```python
from build123d import *

# Parameters (mm, degrees)
SKETCH1_R           = 7.5
BOSS_EXTRUDE1_DEPTH = 46
SKETCH2_W           = 15
SKETCH2_H           = 15
BOSS_EXTRUDE2_DEPTH = 10
BOSS_EXTRUDE3_DEPTH = 15
CUT_EXTRUDE4_DEPTH  = 64.263338514
SKETCH6_R           = 6
CUT_EXTRUDE5_DEPTH  = 64.263338514
SKETCH7_R           = 6
CUT_EXTRUDE6_DEPTH  = 5
CUT_EXTRUDE7_START  = -5
CUT_EXTRUDE7_DEPTH  = 5
SKETCH11_R          = 3.25
SKETCH11_R_2        = 2.25
BOSS_EXTRUDE4_DEPTH = 2.5
BOSS_EXTRUDE5_DEPTH = 2.5


with BuildPart() as part:
    # Sketch1 → Boss-Extrude1 (new body)
    with BuildSketch(Plane(origin=(0, 0, 0), x_dir=(1, 0, 0), z_dir=(0, 1, 0))):
        with Locations(Location((0, 0, 0), (0, 0, 270))):
            Circle(SKETCH1_R)
    extrude(amount=BOSS_EXTRUDE1_DEPTH)

    # Sketch2 → Boss-Extrude2 (add)
    with BuildSketch(Plane.XZ):
        Rectangle(SKETCH2_W, SKETCH2_H)
    extrude(amount=BOSS_EXTRUDE2_DEPTH)

    # Sketch4 → Boss-Extrude3 (add)
    with BuildSketch(Plane(origin=(0, 46, 0), x_dir=(1, 0, 0), z_dir=(0, 1, 0))):
        Polygon((0, 7.5), (7.5, 7.5), (7.5, -7.5), (-7.5, -7.5), (-7.5, 7.5), align=None)
    extrude(amount=BOSS_EXTRUDE3_DEPTH)

    # Sketch5 → Cut-Extrude4 (cut, through all)
    with BuildSketch(Plane.ZY.offset(7.5)):
        with BuildLine():
            ThreePointArc((-7.5, 53.5), (-5.303300859, 58.803300859), (0, 61))
            Line((0, 61), (-7.5, 61))
            Line((-7.5, 61), (-7.5, 53.5))
        make_face()
        with BuildLine():
            Line((7.5, 61), (0, 61))
            ThreePointArc((0, 61), (5.303300859, 58.803300859), (7.5, 53.5))
            Line((7.5, 53.5), (7.5, 61))
        make_face()
    extrude(amount=-CUT_EXTRUDE4_DEPTH, mode=Mode.SUBTRACT)

    # Sketch6 → Cut-Extrude5 (cut, through all)
    with BuildSketch(Plane.ZY.offset(7.5)):
        with Locations((0, 53.5)):
            Circle(SKETCH6_R)
    extrude(amount=-CUT_EXTRUDE5_DEPTH, mode=Mode.SUBTRACT)

    # Sketch7 → Cut-Extrude6 (cut)
    # profile 1 of 4: a face of its own
    with BuildSketch(Plane.ZY.offset(7.5)):
        with BuildLine():
            ThreePointArc((0, 46), (-5.303300859, 48.196699141), (-7.5, 53.5))
            Line((-7.5, 53.5), (-7.5, 46))
            Line((-7.5, 46), (0, 46))
        make_face()
    # profile 2 of 4: a face of its own
    with BuildSketch(Plane.ZY.offset(7.5)):
        with BuildLine():
            Line((7.5, 46), (7.5, 53.5))
            ThreePointArc((7.5, 53.5), (5.303300859, 48.196699141), (0, 46))
            Line((0, 46), (7.5, 46))
        make_face()
    # profile 3 of 4: a face of its own
    with BuildSketch(Plane.ZY.offset(7.5)):
        with BuildLine():
            ThreePointArc((7.5, 53.5), (0, 61), (-7.5, 53.5))
            ThreePointArc((-7.5, 53.5), (-5.303300859, 48.196699141), (0, 46))
            ThreePointArc((0, 46), (5.303300859, 48.196699141), (7.5, 53.5))
        make_face()
        with Locations((0, 53.5)):
            Circle(SKETCH7_R, mode=Mode.SUBTRACT)
    # profile 4 of 4: a face of its own
    with BuildSketch(Plane.ZY.offset(7.5)):
        with Locations((0, 53.5)):
            Circle(SKETCH7_R)
    extrude(amount=-CUT_EXTRUDE6_DEPTH, mode=Mode.SUBTRACT)

    # Sketch10 → Cut-Extrude7 (cut)
    with BuildSketch(Plane(origin=(7.5, 0, 0), x_dir=(0, 0, -1), z_dir=(1, 0, 0)).offset(CUT_EXTRUDE7_START)):
        with BuildLine():
            Line((7.5, 53.5), (6, 53.5))
            ThreePointArc((6, 53.5), (0, 47.5), (-6, 53.5))
            Line((-6, 53.5), (-7.5, 53.5))
            Line((-7.5, 53.5), (-7.5, 46))
            Line((-7.5, 46), (0, 46))
            Line((0, 46), (7.5, 46))
            Line((7.5, 46), (7.5, 53.5))
        make_face()
        with BuildLine():
            ThreePointArc((-6, 53.5), (0, 59.5), (6, 53.5))
            Line((6, 53.5), (7.5, 53.5))
            ThreePointArc((7.5, 53.5), (0, 61), (-7.5, 53.5))
            Line((-7.5, 53.5), (-6, 53.5))
        make_face()
    extrude(amount=CUT_EXTRUDE7_DEPTH, mode=Mode.SUBTRACT)

    # Sketch11 → Boss-Extrude4 (add, symmetric)
    # profile 1 of 3: a face of its own
    with BuildSketch(Plane(origin=(0, 0, 0), x_dir=(-1, 0, 0), z_dir=(0, 0, -1))):
        with BuildLine():
            Line((7.5, -1.75), (7.5, -5))
            ThreePointArc((7.5, -5), (8.451902961, -2.701902961), (10.75, -1.75))
            Line((10.75, -1.75), (7.5, -1.75))
        make_face()
    # profile 2 of 3: a face of its own
    with BuildSketch(Plane(origin=(0, 0, 0), x_dir=(-1, 0, 0), z_dir=(0, 0, -1))):
        with BuildLine():
            Line((7.5, -5), (7.5, -8.25))
            Line((7.5, -8.25), (10.75, -8.25))
            ThreePointArc((10.75, -8.25), (8.451902961, -7.298097039), (7.5, -5))
        make_face()
    # profile 3 of 3: a face of its own
    with BuildSketch(Plane(origin=(0, 0, 0), x_dir=(-1, 0, 0), z_dir=(0, 0, -1))):
        with Locations((10.75, -5)):
            Circle(SKETCH11_R)
        with Locations((10.75, -5)):
            Circle(SKETCH11_R_2, mode=Mode.SUBTRACT)
    extrude(amount=BOSS_EXTRUDE4_DEPTH, both=True)

    # Sketch12 → Boss-Extrude5 (add, symmetric)
    with BuildSketch(Plane(origin=(0, 0, 0), x_dir=(-1, 0, 0), z_dir=(0, 0, -1))):
        with BuildLine():
            Line((-7.5, -8.25), (-7.5, -5))
            ThreePointArc((-7.5, -5), (-8.451902961, -7.298097039), (-10.75, -8.25))
            Line((-10.75, -8.25), (-7.5, -8.25))
        make_face()
        with BuildLine():
            Line((-7.5, -5), (-7.5, -1.75))
            Line((-7.5, -1.75), (-10.75, -1.75))
            ThreePointArc((-10.75, -1.75), (-8.451902961, -2.701902961), (-7.5, -5))
        make_face()
        with BuildLine():
            ThreePointArc((-7.5, -5), (-8.451902961, -2.701902961), (-10.75, -1.75))
            Line((-10.75, -1.75), (-10.75, -2.75))
            ThreePointArc((-10.75, -2.75), (-9.159009742, -3.409009742), (-8.5, -5))
            Line((-8.5, -5), (-7.5, -5))
        make_face()
        with BuildLine():
            ThreePointArc((-10.75, -8.25), (-8.451902961, -7.298097039), (-7.5, -5))
            Line((-7.5, -5), (-8.5, -5))
            ThreePointArc((-8.5, -5), (-9.159009742, -6.590990258), (-10.75, -7.25))
            Line((-10.75, -7.25), (-10.75, -8.25))
        make_face()
        with BuildLine():
            Line((-10.75, -2.75), (-10.75, -1.75))
            ThreePointArc((-10.75, -1.75), (-14, -5), (-10.75, -8.25))
            Line((-10.75, -8.25), (-10.75, -7.25))
            ThreePointArc((-10.75, -7.25), (-13, -5), (-10.75, -2.75))
        make_face()
    extrude(amount=BOSS_EXTRUDE5_DEPTH, both=True)


solid = part.part
```
Geometry check sheet. Reference: the model listing, model coordinates, mm. A direction names the side the tool comes from. Coordinates: 2 decimals unless noted, no trailing zeros. Order: outer loops, then holes, each group sorted by start corner. A loop starts at its lowest first (then second) coordinate and runs counter-clockwise, first axis right, second up. Notation, with made-up numbers: (32.5, 78) - (68.5, 78) arc R20 cw to (68.5, 97) - close; hole circle Ø10 at (72, -37.75). An arc over 180 degrees is marked (long way). Answer as a JSON object with one key per item and string values. Group by question number.
Item 1: Sectioned sample at D-D, the plane x = 4.25. Record the cut outline in (y, z).
Item 2: Sectioned sample at A-A, the plane x = 1.25. Record the cut outline in (y, z).
Item 3: Sectioned sample at C-C, the plane y = 18.5. Record the cut outline in (x, z).
Item 4: Tool access check on faces 1 (the face through (9, -1.75, 0)), 2 (the face through (-8.5, -3.5, 2.5)), 3 (the face through (-4, 46, 0)), 4 (the face through (-8.5, -3.5, -2.5)), 5 (the face through (9, -8.25, 0)). Record the directions out of +Z, -Z, +X, -X, +Y, -Y that give a thin tool (end or side, any length) a straight path to the whole face; none if there is none.
Item 5: Depth check by flat-ended pin: pin 1 Ø8 at (x, z) = (-5.5, -4) entering from +Y; pin 2 Ø1.6 at (x, z) = (9.5, 0.5) entering from -Y; pin 3 Ø8 at (x, y) = (5, 35.5) entering from +Z. Enter the tip coordinate at first touch or a pass-through.
Item 6: Sectioned sample at B-B, the plane x = -5. Record the cut outline in (y, z).
Item 7: Scan lines: probe 1 along Y at (x, z) = (-0.9, 0); probe 2 along Y at (x, z) = (-10.75, 1.8); probe 3 along X at (y, z) = (43, 2.5). Record each from-to range of solid material in increasing order.
Resolved:
{
 "1": {"outline": "(-10, -7.5) - (0, -7.5) - (0, -6.18) - (46, -6.18) - (46, 6.18) - (0, 6.18) - (0, 7.5) - (-10, 7.5) - close"},
 "2": {"outline": "(-10, -7.5) - (0, -7.5) - (0, -7.4) - (46, -7.4) - (46, -7.5) - (53.5, -7.5) arc R7.5 ccw to (53.5, 7.5) - (46, 7.5) - (46, 7.4) - (0, 7.4) - (0, 7.5) - (-10, 7.5) - close; hole circle Ø12 at (53.5, 0)"},
 "3": {"outline": "circle Ø15 at (0, 0)"},
 "4": {"face 1": "+Z, -Z, +X, +Y", "face 2": "+Z, -X, +Y, -Y", "face 3": "+Z, -Z, -X, +Y", "face 4": "-Z, -X, +Y, -Y", "face 5": "+Z, -Z, +X, -Y"},
 "5": {"pin 1": "y = 60.88", "pin 2": "y = -8.25", "pin 3": "z = 7.43"},
 "6": {"outline": "(-10, -7.5) - (0, -7.5) - (0, -5.59) - (46, -5.59) - (46, 5.59) - (0, 5.59) - (0, 7.5) - (-10, 7.5) - close"},
 "7": {"probe 1": "-10 to 47.5, 59.5 to 61", "probe 2": "-8.25 to -7.25, -2.75 to -1.75", "probe 3": "-7.07 to 7.07"}
}
